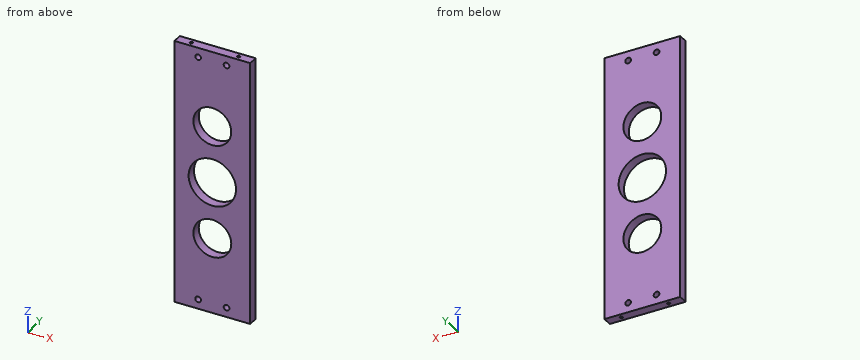
from build123d import *

# Parameters (mm, degrees)
SKETCH1_R           = 3
SKETCH1_R_2         = 25
SKETCH1_R_3         = 20
BOSS_EXTRUDE1_DEPTH = 10
SKETCH2_R           = 1.5
CUT_EXTRUDE1_DEPTH  = 15


with BuildPart() as part:
    # Sketch1 → Boss-Extrude1 (new body)
    with BuildSketch(Plane(origin=(0, 0, 0), x_dir=(1, 0, 0), z_dir=(0, 1, 0))):
        Polygon((0, -110), (0, 110), (0, 140), (80, 140), (80, 110), (80, -110), (80, -140), (0, -140), align=None)
        with Locations(Location((25, 130, 0), (0, 0, 270))):
            Circle(SKETCH1_R, mode=Mode.SUBTRACT)
        with Locations(Location((55, 130, 0), (0, 0, 270))):
            Circle(SKETCH1_R, mode=Mode.SUBTRACT)
        with Locations(Location((25, -130, 0), (0, 0, 270))):
            Circle(SKETCH1_R, mode=Mode.SUBTRACT)
        with Locations(Location((55, -130, 0), (0, 0, 270))):
            Circle(SKETCH1_R, mode=Mode.SUBTRACT)
        with Locations(Location((40, 0, 0), (0, 0, 270))):
            Circle(SKETCH1_R_2, mode=Mode.SUBTRACT)
        with Locations(Location((40, -60, 0), (0, 0, 270))):
            Circle(SKETCH1_R_3, mode=Mode.SUBTRACT)
        with Locations(Location((40, 60, 0), (0, 0, 270))):
            Circle(SKETCH1_R_3, mode=Mode.SUBTRACT)
    extrude(amount=BOSS_EXTRUDE1_DEPTH)

    # Sketch2 → Cut-Extrude1 (cut)
    with BuildSketch(Plane.XY.offset(140)):
        with Locations((15, 5)):
            Circle(SKETCH2_R)
        with Locations((65, 5)):
            Circle(SKETCH2_R)
    cut_extrude1 = extrude(amount=-CUT_EXTRUDE1_DEPTH, mode=Mode.SUBTRACT)

    # Mirror1: Cut-Extrude1 across plane
    add(cut_extrude1.mirror(Plane.XY), mode=Mode.SUBTRACT)


solid = part.part
The listing builds one solid part. Answer for the finished solid, in the listing's coordinates (mm). Round coordinates to 2 decimals unless told otherwise and drop trailing zeros. Write each loop counter-clockwise with the first axis right and the second up, starting at its lowest first coordinate (ties: lowest second). Pieces come first, ordered by that corner, then holes. Notation, with made-up numbers: (3.5, -38) - (51.5, -38) arc R37 cw to (51.5, 0) - close; hole circle Ø2 at (7, -23.5). An arc over 180 degrees is marked (long way). Use a Markdown table: item, result. Add a question column.
1. Consider line 1 (Z direction, x = 41, y = 8.75); line 2 (X direction, y = 3.75, z = -130); line 3 (X direction, y = 6.75, z = 58.5). Determine where each line is inside the solid, lowest interval first.
2. The part is cut by section A-A (y = 5). Write down the section's boundary in (x, z).
3. Flat-ended cylindrical pins translate along their axes: P1, Ø0.9, axis at x = 65, y = 5, coming from the -Z side; P2, Ø1.5, axis at x = 14.5, y = 5.5, coming from the +Z side. Find the tip coordinate at first contact, or state that the pin passes through.
4. The part is cut by section B-B (z = -130). Write down the section's boundary in (x, y).
5. The part is cut by section C-C (x = 45). Write down the section's boundary in (y, z), and give its area (3 significant figures).
6. The part is cut by section D-D (z = 60). Write down the section's boundary in (x, y), and give its area (3 significant figures).
Reported:
| question | item | result |
|---|---|---|
| 1 | line 1 | -140 to -79.97, -40.03 to -24.98, 24.98 to 40.03, 79.97 to 140 |
| 1 | line 2 | 0 to 14.17, 15.83 to 22, 28 to 52, 58 to 64.17, 65.83 to 80 |
| 1 | line 3 | 0 to 20.06, 59.94 to 80 |
| 2 | outline | (0, -140) - (13.5, -140) - (13.5, -125) - (16.5, -125) - (16.5, -140) - (63.5, -140) - (63.5, -125) - (66.5, -125) - (66.5, -140) - (80, -140) - (80, 140) - (66.5, 140) - (66.5, 125) - (63.5, 125) - (63.5, 140) - (16.5, 140) - (16.5, 125) - (13.5, 125) - (13.5, 140) - (0, 140) - close; hole circle Ø50 at (40, 0); hole circle Ø40 at (40, -60); hole circle Ø40 at (40, 60); hole circle Ø6 at (25, -130); hole circle Ø6 at (25, 130); hole circle Ø6 at (55, -130); hole circle Ø6 at (55, 130) |
| 3 | P1 | z = -125 |
| 3 | P2 | z = 125 |
| 4 | outline | (0, 0) - (22, 0) - (22, 10) - (0, 10) - close; (28, 0) - (52, 0) - (52, 10) - (28, 10) - close; (58, 0) - (80, 0) - (80, 10) - (58, 10) - close; hole circle Ø3 at (15, 5); hole circle Ø3 at (65, 5) |
| 5 | outline | (0, -140) - (10, -140) - (10, -79.36) - (0, -79.36) - close; (0, -40.64) - (10, -40.64) - (10, -24.49) - (0, -24.49) - close; (0, 24.49) - (10, 24.49) - (10, 40.64) - (0, 40.64) - close; (0, 79.36) - (10, 79.36) - (10, 140) - (0, 140) - close |
| 5 | area | 1,540 mm^2 |
| 6 | outline | (0, 0) - (20, 0) - (20, 10) - (0, 10) - close; (60, 0) - (80, 0) - (80, 10) - (60, 10) - close |
| 6 | area | 400 mm^2 |
